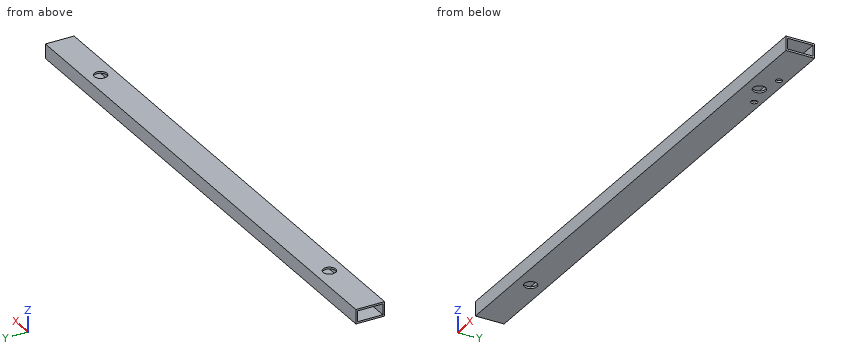
Autodesk Inventor part; units mm, degrees
ref_plane "YZ Plane" through (0, 0, 0) normal (1, 0, 0) x (0, 1, 0)
ref_plane "XZ Plane" through (0, 0, 0) normal (0, 1, 0) x (-1, 0, 0)
ref_plane "XY Plane" through (0, 0, 0) normal (0, 0, 1) x (1, 0, 0)
sketch "Sketch1" plane through (0, 0, 0) normal (0, 0, 1) x (1, 0, 0)
  line L0 (0, 0) -> (-965.2, 0)
  line L1 (-965.2, 0) -> (-965.2, 50.8)
  line L2 (-965.2, 50.8) -> (0, 50.8)
  line L3 (0, 50.8) -> (0, 0)
  dimension "d0" = 50.8
  dimension "d1" = 965.2
extrude "Extrusion1" add sketch "Sketch1" along normal blind 25.4
sketch "Sketch2" plane through (0, 0, 0) normal (1, 0, 0) x (0, 0, -1)
  line L0 (-3.175, 3.175) -> (-22.225, 3.175)
  line L1 (-22.225, 3.175) -> (-22.225, 47.625)
  line L2 (-22.225, 47.625) -> (-3.175, 47.625)
  line L3 (-3.175, 47.625) -> (-3.175, 3.175)
  line L4 (0, 0) -> (-25.4, 0)
  line L5 (0, 50.8) -> (0, 0)
  line L6 (0, 50.8) -> (-25.4, 50.8)
  line L7 (-25.4, 0) -> (-25.4, 50.8)
  dimension "d5" = 3.175
  dimension "d7" = 3.175
  dimension "d8" = 3.175
  dimension "d9" = 3.175
extrude "Extrusion2" cut sketch "Sketch2" against normal blind 965.2 contours L0 L1 L2 L3
sketch "Sketch3" plane through (0, 0, 25.4) normal (0, 0, 1) x (1, 0, 0)
  circle A0 centre (-838.2, 25.4) radius 6.2992
  line L0 (-965.2, 0) -> (0, 0)
  line L1 (-965.2, 0) -> (0, 0)
  line L2 (-965.2, 50.8) -> (-965.2, 0)
  line L3 (0, 0) -> (0, 50.8)
  circle A1 centre (-127, 25.4) radius 11.1125
  dimension "d13" = 25.4
  dimension "d14" = 12.5984
  dimension "d16" = 127
  dimension "d18" = 22.225
hole "Hole1" at (-838.2, 25.4, 25.4) at (-127, 25.4, 25.4) direction (0, 0, -1) diameter 22.225 end through all
sketch "Sketch4" plane through (0, 0, 0) normal (0, 0, -1) x (-1, 0, 0)
  circle A0 centre (165.735, 38.2537) radius 5.5563
  arc A1 (85.416, 33.4832) -> (85.0155, 42.761) centre (88.5446, 38.2658) ccw
  arc A2 (85.0155, 42.761) -> (85.416, 33.4832) centre (88.265, 38.2537) ccw
  circle A3 centre (165.735, 38.2537) radius 5.5563
  circle A4 centre (88.265, 38.2537) radius 5.5565
  point P0 (0, 0)
extrude "Extrusion3" cut sketch "Sketch4" against normal blind 5.08 contours A0 | A2 A4
The listing builds one solid part. Answer for the finished solid, in the listing's coordinates (mm). Give positions to 0.01 mm unless a question says otherwise; leave off trailing zeros. Write each loop counter-clockwise with the first axis right and the second up, starting at its lowest first coordinate (ties: lowest second). Pieces come first, ordered by that corner, then holes.
1) Find the intervals of material crossed by L1, parallel to X at y = 25.4, z = 0.8; L2, parallel to Z at x = -448, y = 4.5 (3 decimals); L3, parallel to Y at x = -581.5, z = 16 (3 decimals), in increasing order.
2) Section A-A (x = -127) is taken. Write down the section's boundary in (y, z) (1 decimal), and give its area (3 significant figures).
3) Given P1, Ø15, axis at x = -279.5, z = 13, coming from the -Y side, flat-ended and moving along its own axis, determine where the tip first touches the part or whether it passes through.
4) Section B-B (z = 8.75) is taken. Write down the section's boundary in (x, y) (3 decimals), and give its area (3 significant figures).
5) Section C-C (x = -290) is taken. Write down the section's boundary in (y, z) (3 decimals), and give its area (3 significant figures).
Response:
1. L1: x = -965.2 to -849.31, -827.09 to -138.11, -115.89 to 0
1. L2: z = 0 to 3.175, 22.225 to 25.4
1. L3: y = 0 to 3.175, 47.625 to 50.8
2. outline: (0, 0) - (14.3, 0) - (14.3, 3.2) - (3.2, 3.2) - (3.2, 22.2) - (14.3, 22.2) - (14.3, 25.4) - (0, 25.4) - close; (36.5, 0) - (50.8, 0) - (50.8, 25.4) - (36.5, 25.4) - (36.5, 22.2) - (47.6, 22.2) - (47.6, 3.2) - (36.5, 3.2) - close
2. area: 302 mm2
3. P1: stops at y = 0
4. outline: (-965.2, 0) - (0, 0) - (0, 3.175) - (-965.2, 3.175) - close; (-965.2, 47.625) - (0, 47.625) - (0, 50.8) - (-965.2, 50.8) - close
4. area: 6,130 mm2
5. outline: (0, 0) - (50.8, 0) - (50.8, 25.4) - (0, 25.4) - close; hole (3.175, 3.175) - (47.625, 3.175) - (47.625, 22.225) - (3.175, 22.225) - close
5. area: 444 mm2
